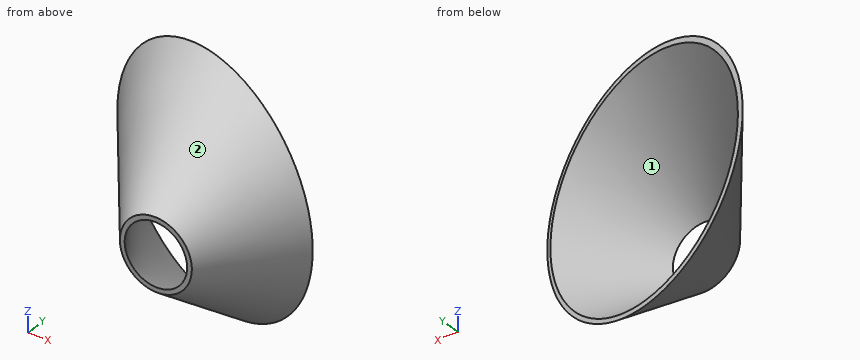
from build123d import *

# Parameters (mm, degrees)
SHELL1_T                = -2.54
CUT_EXTRUDE4_DEPTH      = 176.976362049
CUT_EXTRUDE4_DEPTH_BACK = 176.976362049


with BuildPart() as part:
    # Sketch3 → Revolve1 (revolve)
    with BuildSketch(Plane.XY, mode=Mode.PRIVATE) as revolve1_sk:
        Polygon((0, 0), (-24.257, 0), (-101.6, 101.6), (0, 101.6), align=None)
    revolve(revolve1_sk.sketch.rotate(Axis((0, 0, 0), (0, 1, 0)), 90), axis=Axis((0, 0, 0), (0, 1, 0)))

    # Shell1
    shell1_openings = [part.faces().sort_by_distance(p)[0] for p in [
        (0, 101.6, 0),
        (0, 0, 0),
    ]]
    offset(amount=SHELL1_T, openings=shell1_openings, kind=Kind.INTERSECTION)

    # Sketch4 → Cut-Extrude4 (cut, two sides: drawn at the far end of the back side and taken through both)
    with BuildSketch(Plane.XY.offset(-CUT_EXTRUDE4_DEPTH_BACK)):
        Polygon((101.6, 101.6), (0, 101.6), (-101.6, 101.6), (65.441557357, 54.101224771), align=None)
    extrude(amount=CUT_EXTRUDE4_DEPTH + CUT_EXTRUDE4_DEPTH_BACK, mode=Mode.SUBTRACT)


solid = part.part
Could you check a few things on this model? Use its own coordinates, in mm. Face numbers are marked on the shaded views. Round coordinates to 2 decimals unless told otherwise and drop trailing zeros. Write each loop counter-clockwise with the first axis right and the second up, starting at its lowest first coordinate (ties: lowest second). Pieces come first, ordered by that corner, then holes. Notation, with made-up numbers: (-34, 69) - (2, 69) arc R23 cw to (2, 93) - close; hole circle Ø1 at (33.25, 33). An arc over 180 degrees is marked (long way). Put each result on its own line as item: value. Start each with the question number.
(1) Will these pins go through, and if not, where does the flat tip stop? pin 1 (10 mm diameter, centred on x = -66.5, z = -30, fed in from +Y); pin 2 (1 mm diameter, centred on x = 2.5, y = 53.5, fed in from -Z); pin 3 (4 mm diameter, centred on y = 71, z = -30.5, fed in from +X).
(2) Thinking about a two-plate mould opening in X: for the marked faces 1 and 2, which applies, released by +X, released by -X, zero draft, split by the parting line, or undercut?
(3) I want a section at A-A, the plane x = 0. Please give me the cut outline in (y, z).
(4) I need wall thicknesses on probe 1 along Z at (x, y) = (-54, 82.5); probe 2 along Z at (x, y) = (13, 23.5); probe 3 along X at (y, z) = (30.5, -38). Which ranges of each line are inside material? Lowest first, please.
(5) I want a section at C-C, the plane y = 20.5. Please give me the cut outline in (x, z), plus the area to 3 significant figures.
(6) I want a section at B-B, the plane y = 32. Please give me the cut outline in (x, z).
Here are the results:
1. pin 1: stops at y = 74.73
1. pin 2: stops at z = -65.32
1. pin 3: stops at x = -66.73
2. face 1: undercut
2. face 2: split by the parting line
3. outline: (0, -24.26) - (72.71, -79.61) - (72.71, -76.42) - (0, -21.06) - close; (0, 21.06) - (72.71, 76.42) - (72.71, 79.61) - (0, 24.26) - close
4. probe 1: z = -68.29 to -64.17, 64.17 to 68.29
4. probe 2: z = -40.09 to -36.72, 36.72 to 40.09
4. probe 3: x = -28.46 to -22.74, 22.74 to 28.46
5. outline: circle Ø79.73 at (0, 0); hole circle Ø73.34 at (0, 0)
5. area: 768 mm^2
6. outline: circle Ø97.23 at (0, 0); hole circle Ø90.85 at (0, 0)
